Geometry: final body of the model. Coordinates: model frame, mm. Face numbers are marked on the shaded views. A direction names the side the tool comes from. Give positions to 0.01 mm unless a question says otherwise; leave off trailing zeros. Write each loop counter-clockwise with the first axis right and the second up, starting at its lowest first coordinate (ties: lowest second). Pieces come first, ordered by that corner, then holes. Notation, with made-up numbers: M 18,46.25 L 49,46.25 A29 ccw 49,76.25 Z; hole C -12,-11 d11. An arc over 180 degrees is marked long. One line per question, with ' | ' between items.
from build123d import *

# Parameters (mm, degrees)
SKETCH1_R           = 44.5
BOSS_EXTRUDE1_DEPTH = 2.5
SKETCH2_R           = 1.5
CUT_EXTRUDE1_DEPTH  = 63.982140326
SKETCH3_R           = 35.5
BOSS_EXTRUDE2_DEPTH = 20
SKETCH4_R           = 33.75
BOSS_EXTRUDE3_DEPTH = 28.5


with BuildPart() as part:
    # Sketch1 → Boss-Extrude1 (new body)
    with BuildSketch(Plane.XY):
        Circle(SKETCH1_R)
    extrude(amount=BOSS_EXTRUDE1_DEPTH)

    # Sketch2 → Cut-Extrude1 (cut, through all)
    with BuildSketch(Plane.XY.offset(2.5)):
        with Locations((0, 41.75)):
            Circle(SKETCH2_R)
        with Locations((41.75, 0)):
            Circle(SKETCH2_R)
        with Locations((0, -41.75)):
            Circle(SKETCH2_R)
        with Locations((-41.75, 0)):
            Circle(SKETCH2_R)
    extrude(amount=-CUT_EXTRUDE1_DEPTH, mode=Mode.SUBTRACT)

    # Sketch3 → Boss-Extrude2 (add)
    with BuildSketch(Plane.XY.offset(2.5)):
        Circle(SKETCH3_R)
    extrude(amount=BOSS_EXTRUDE2_DEPTH)

    # Sketch4 → Boss-Extrude3 (add)
    with BuildSketch(Plane.XY.offset(22.5)):
        with Locations(Location((0, 0, 0), (0, 0, 180))):
            Circle(SKETCH4_R)
    extrude(amount=BOSS_EXTRUDE3_DEPTH)


solid = part.part
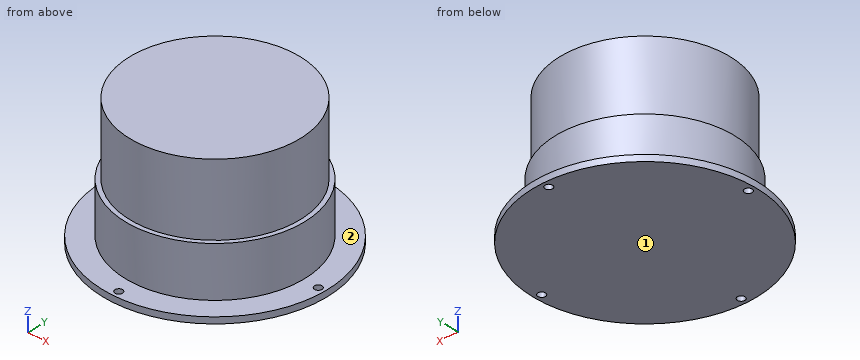
(1) Material intervals for L1, parallel to Y at x = 0, z = 1; L2, parallel to Z at x = 32, y = 30.5; L3, parallel to X at y = 5.5, z = 19.5, sorted ascending. Write a range as [from, to].
Working result:
L1: y = [-44.5, -43.25], [-40.25, 40.25], [43.25, 44.5] | L2: z = [0, 2.5] | L3: x = [-35.07, 35.07]
(2) Set-up query: the marked faces 1 and 2. Return all of +Z, -Z, +X, -X, +Y, -Y with unobstructed straight access to the full face (end or side cutting, diameter ignored); none if empty.
Working result:
face 1: -Z, +X, -X, +Y, -Y | face 2: +Z
(3) First-contact query: P1, Ø1.5, axis at y = 13.5, z = 40.5, coming from the -X side; P2, Ø1.5, axis at y = -22.5, z = 32.5, coming from the +X side; P3, Ø8, axis at x = 0, z = 45, coming from the +Y side. Flat tips, straight axial feed; report the tip coordinate or a pass-through.
Working result:
P1: stops at x = -31.25 | P2: stops at x = 25.81 | P3: stops at y = 33.75
(4) Cut plane D-D, the plane z = 15.5. Return loops of the section in (x, y).
Working result:
outline: C 0,0 d71
(5) Cut plane A-A, the plane y = 0. Return loops of the section in (x, z), then the cut area to 3 significant figures.
Working result:
outline: M -44.5,0 L -43.25,0 L -43.25,2.5 L -44.5,2.5 Z; M -40.25,0 L 40.25,0 L 40.25,2.5 L 35.5,2.5 L 35.5,22.5 L 33.75,22.5 L 33.75,51 L -33.75,51 L -33.75,22.5 L -35.5,22.5 L -35.5,2.5 L -40.25,2.5 Z; M 43.25,0 L 44.5,0 L 44.5,2.5 L 43.25,2.5 Z | area: 3,550 mm^2
(6) Cut plane C-C, the plane y = 41.75. Return loops of the section in (x, z), then the cut area to 3 significant figures.
Working result:
outline: M -15.4,0 L -1.5,0 L -1.5,2.5 L -15.4,2.5 Z; M 1.5,0 L 15.4,0 L 15.4,2.5 L 1.5,2.5 Z | area: 69.5 mm^2
